Build history of the part. All positions in model axes, mm. A direction names the side the tool comes from. Round coordinates to 2 decimals unless told otherwise and drop trailing zeros. Order: outer loops, then holes, each group sorted by start corner. A loop starts at its lowest first (then second) coordinate and runs counter-clockwise, first axis right, second up. Notation, with made-up numbers: M -38,22 L 9,22 A8 ccw 9,29 Z; hole C 53.5,39 d11. An arc over 180 degrees is marked long. One line per item, written item: value. Start each with the question number.
Item 1: Probe L1, parallel to Z at x = 0, y = -4.5 (3 decimals); L2, parallel to X at y = -3.5, z = 4 (1 decimal); L3, parallel to Y at x = -20.5, z = 41.5. List the from-to ranges inside material, lowest first.
Item 2: Band-saw the part on A-A, the plane x = 0. Write the cut outline in (y, z) (3 decimals).
Item 3: Tool access for faces 4 (the cylindrical face through (24.384, -9.481, 2.48)), 5 (the flat face through (4.762, -3, 0)), 6 (the flat face through (0, -3, 60.325)): list every direction of +Z, -Z, +X, -X, +Y, -Y with a clear straight run to the whole face (end or side of a thin tool).
Item 4: Two-plate mould, pull along Z, no slides. Class faces 1 (the flat face through (16, -12.7, -2)), 2 (the cylindrical face through (14.924, -6.261, 0.07)), 3 (the cylindrical face through (-23.061, -9.481, -5.023)): +Z half, -Z half, draft (parallel to the pull), parting line (faces both ways), or undercut.
Item 5: Band-saw the part on B-B, the plane z = 0. Give the number of separate pieces and of enclosed holes in the cut face, then the cut area to 3 significant figures.
Item 6: Pin check, flat tips, straight feed: pin 1 (6 mm diameter, centred on x = 3.5, z = 38.5, fed in from -Y); pin 2 (6 mm diameter, centred on y = -11, z = -42, fed in from +X). Stop position of each tip, or through.
Item 7: Band-saw the part on D-D, the plane y = -8. Write the cut outline in (x, z) (1 decimal).
```python
from build123d import *

# Parameters (mm, degrees)
F0_W     = 69.85
F0_H     = 120.65
F0_R     = 1.5875
F0_R_2   = 8.255
F0_W_2   = 9.525
F0_H_2   = 25.4
F1_DEPTH = 6.35
F2_DEPTH = 12.7
F3_DEPTH = 12.7


with BuildPart() as f1:
    # F0 (on Front) → F1 (new body)
    with BuildSketch(Plane.XZ):
        Rectangle(F0_W, F0_H)
        with Locations((0, -29.0322)):
            Circle(F0_R, mode=Mode.SUBTRACT)
        with Locations((-16.51, 0)):
            Circle(F0_R_2, mode=Mode.SUBTRACT)
        Rectangle(F0_W_2, F0_H_2, mode=Mode.SUBTRACT)
        with Locations((16.51, 0)):
            Circle(F0_R_2, mode=Mode.SUBTRACT)
        with Locations((0, 29.028019)):
            Circle(F0_R, mode=Mode.SUBTRACT)
    extrude(amount=F1_DEPTH)

    # F0 (on Front) → F2 (join)
    with BuildSketch(Plane.XZ):
        with Locations((-16.51, 0)):
            Circle(F0_R_2)
        with Locations((-16.51, 0)):
            Circle(F0_R, mode=Mode.SUBTRACT)
    extrude(amount=F2_DEPTH)

    # F0 (on Front) → F3 (join)
    with BuildSketch(Plane.XZ):
        with Locations((16.51, 0)):
            Circle(F0_R_2)
        with Locations((16.51, 0)):
            Circle(F0_R, mode=Mode.SUBTRACT)
    extrude(amount=F3_DEPTH)


solid = f1.part
```
Output:
1. L1: z = -60.325 to -30.62, -27.445 to -12.7, 12.7 to 27.441, 30.616 to 60.325
1. L2: x = -34.9 to -4.8, 4.8 to 34.9
1. L3: y = -6.35 to 0
2. outline: M -6.35,-60.325 L 0,-60.325 L 0,-30.62 L -6.35,-30.62 Z; M -6.35,-27.445 L 0,-27.445 L 0,-12.7 L -6.35,-12.7 Z; M -6.35,12.7 L 0,12.7 L 0,27.441 L -6.35,27.441 Z; M -6.35,30.616 L 0,30.616 L 0,60.325 L -6.35,60.325 Z
3. face 4: -Y
3. face 5: +Y, -Y
3. face 6: +Z, +X, -X, +Y, -Y
4. face 1: draft
4. face 2: undercut
4. face 3: parting line
5. separate pieces: 4
5. enclosed holes: 0
5. area: 512 mm²
6. pin 1: stops at y = -6.35
6. pin 2: passes through
7. outline: C -16.5,0 d16.5; C 16.5,0 d16.5; hole C -16.5,0 d3.2; hole C 16.5,0 d3.2
